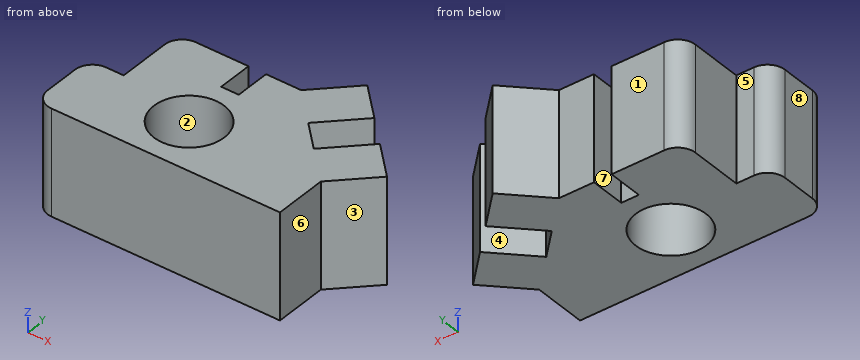
```python
from build123d import *

# Parameters (mm, degrees)
F0_R     = 10
F1_DEPTH = 30


with BuildPart() as f1:
    # F0 (on Top) → F1 (new body)
    with BuildSketch(Plane.XY):
        with BuildLine():
            ThreePointArc((-24.06338, -22.053742), (-22.598914, -25.589276), (-19.06338, -27.053742))
            Line((-19.06338, -27.053742), (45.93662, -27.053742))
            Line((45.93662, -27.053742), (45.93662, -12.053742))
            Line((45.93662, -12.053742), (56.543221, -1.44714))
            Line((56.543221, -1.44714), (47.578755, 7.517326))
            Line((47.578755, 7.517326), (36.972154, -3.089276))
            Line((36.972154, -3.089276), (29.901086, 3.981792))
            Line((29.901086, 3.981792), (40.507688, 14.588394))
            Line((40.507688, 14.588394), (31.543221, 23.55286))
            Line((31.543221, 23.55286), (20.93662, 12.946258))
            Line((20.93662, 12.946258), (10.93662, 12.946258))
            Line((10.93662, 12.946258), (10.93662, 2.946258))
            Line((10.93662, 2.946258), (5.93662, 2.946258))
            Line((5.93662, 2.946258), (5.93662, 12.946258))
            Line((5.93662, 12.946258), (-9.06338, 12.946258))
            ThreePointArc((-9.06338, 12.946258), (-12.598914, 11.481792), (-14.06338, 7.946258))
            Line((-14.06338, 7.946258), (-14.06338, -7.053742))
            Line((-14.06338, -7.053742), (-19.06338, -7.053742))
            ThreePointArc((-19.06338, -7.053742), (-22.598914, -8.518208), (-24.06338, -12.053742))
            Line((-24.06338, -12.053742), (-24.06338, -22.053742))
        make_face()
        with Locations((8.43662, -12.053742)):
            Circle(F0_R, mode=Mode.SUBTRACT)
    extrude(amount=F1_DEPTH)


solid = f1.part
```
CAD build for the part. Positions are in the model's coordinates, mm. Face numbers are marked on the shaded views. A direction names the side the tool comes from. Round coordinates to 2 decimals unless told otherwise and drop trailing zeros. Order: outer loops, then holes, each group sorted by start corner. A loop starts at its lowest first (then second) coordinate and runs counter-clockwise, first axis right, second up.
Item 1: Saw through at D-D on x = -4. Write the cut outline in (y, z), then the cut area to 3 significant figures.
Item 2: Tool access for the marked faces 4, 5, 6, 7 and 8: list every direction of +Z, -Z, +X, -X, +Y, -Y with a clear straight run to the whole face (end or side of a thin tool).
Item 3: Saw through at A-A on y = -20.5. Write the cut outline in (x, z), then the cut area to 3 significant figures.
Item 4: Mould opens along Y. For the marked faces 1, 2 and 3 say: pulls with the +Y half, pulls with the -Y half, needs draft (parallel to the pull), parting line crosses it, or undercut.
Item 5: Saw through at C-C on y = 9.5. Write the cut outline in (x, z).
Item 6: Pin check, flat tips, straight feed: pin 1 (8 mm diameter, centred on x = 20.5, z = 19, fed in from +Y); pin 2 (5.5 mm diameter, centred on x = 8.5, z = 14.5, fed in from +Y); pin 3 (4 mm diameter, centred on y = 18, z = 11, fed in from +X). Stop position of each tip, or through.
Item 7: Probe line 1 along X through (y, z) = (5, 20.75); line 2 along Y through (x, z) = (20, 4); line 3 along X through (y, z) = (-3, 13). List the from-to ranges inside material, lowest first.
Item 8: Saw through at B-B on z = 24. Write the cut outline in (x, y), then the cut area to 3 significant figures.
Reported:
1. outline: (-27.05, 0) - (12.95, 0) - (12.95, 30) - (-27.05, 30) - close
1. area: 1,200 mm2
2. face 4: +Z, -Z
2. face 5: +Z, -Z, -X, +Y
2. face 6: +Z, -Z, +X, -Y
2. face 7: +Z, -Z, +Y
2. face 8: +Z, -Z, -X, +Y, -Y
3. outline: (-24.06, 0) - (3.08, 0) - (3.08, 30) - (-24.06, 30) - close; (13.79, 0) - (45.94, 0) - (45.94, 30) - (13.79, 30) - close
3. area: 1,780 mm2
4. face 1: pulls with the +Y half
4. face 2: undercut
4. face 3: pulls with the -Y half
5. outline: (-13.82, 0) - (5.94, 0) - (5.94, 30) - (-13.82, 30) - close; (10.94, 0) - (35.42, 0) - (35.42, 30) - (10.94, 30) - close
6. pin 1: stops at y = 16.51
6. pin 2: stops at y = 12.95
6. pin 3: stops at x = 39.1
7. line 1: x = -14.06 to 5.94, 10.94 to 30.92, 45.06 to 50.1
7. line 2: y = -27.05 to 12.95
7. line 3: x = -14.06 to 4.19, 12.68 to 36.88, 37.06 to 54.99
8. outline: (-24.06, -22.05) arc R5 ccw to (-19.06, -27.05) - (45.94, -27.05) - (45.94, -12.05) - (56.54, -1.45) - (47.58, 7.52) - (36.97, -3.09) - (29.9, 3.98) - (40.51, 14.59) - (31.54, 23.55) - (20.94, 12.95) - (10.94, 12.95) - (10.94, 2.95) - (5.94, 2.95) - (5.94, 12.95) - (-9.06, 12.95) arc R5 ccw to (-14.06, 7.95) - (-14.06, -7.05) - (-19.06, -7.05) arc R5 ccw to (-24.06, -12.05) - close; hole circle Ø20 at (8.44, -12.05)
8. area: 2,290 mm2
